Part model, mm, in its own coordinate system. A direction names the side the tool comes from. Round coordinates to 2 decimals unless told otherwise and drop trailing zeros. Order: outer loops, then holes, each group sorted by start corner. A loop starts at its lowest first (then second) coordinate and runs counter-clockwise, first axis right, second up. Notation, with made-up numbers: M 53.5,67 L 93.5,67 A22 ccw 93.5,86 Z; hole C 89.25,-18 d2. An arc over 180 degrees is marked long. Write each question's results on one line, items separated by ' | '. Start each with the question number.
1. Band-saw the part on A-A, the plane y = 0. List the corners of the cut face in (x, z), then the cut area to 3 significant figures.
2. Band-saw the part on D-D, the plane z = 13.5. List the corners of the cut face in (x, y), then the cut area to 3 significant figures.
3. Which spindle directions (+Z, -Z, +X, -X, +Y, -Y) get a long thin tool onto all of the face, cutting with end or side? Do faces 1 (the face through (20.765, 39.923, 49.58)), 2 (the face through (-14.985, -0.66, 29.58)). Say none if no direction does.
4. Two-plate mould, pull along X, no slides. Class faces 3 (the face through (-120, 0, 10)), 4 (the face through (15, -7, 60)), 5 (the face through (120, 0, 10)): +X half, -X half, draft (parallel to the pull), parting line (faces both ways), or undercut.
5. Drop flat-ended pins along their axis: pin 1 Ø12 at (y, z) = (-6.5, 14.5) entering from +X; pin 2 Ø2 at (x, y) = (36, 20) entering from -Z; pin 3 Ø5 at (x, z) = (-15.5, 61) entering from -Y; pin 4 Ø1.5 at (x, z) = (-8.5, 69) entering from +Y. Give the stop position or say it passes through.
6. Band-saw the part on C-C, the plane z = 51.5. List the corners of the cut face in (x, y), then the cut area to 3 significant figures.
7. Probe L1, parallel to Y at x = 0, z = 13; L2, parallel to Y at x = 0, z = 31; L3, parallel to Z at x = -22.5, y = -2. List the from-to ranges inside material, lowest first. Write a range as [from, to].
8. Band-saw the part on B-B, the plane x = -100. List the corners of the cut face in (y, z), then the cut area to 3 significant figures.
Autodesk Fusion 360 part; units mm, degrees
sketch "Sketch1" plane through (0, 0, 0) normal (0, 0, 1) x (1, 0, 0)
  circle A0 centre (0, 0) radius 15
  circle A1 centre (0, 0) radius 35
  circle A2 centre (0, 0) radius 45
  line L0 (-100, -20.9657) -> (-100, -80.0578) construction
  circle A3 centre (-100, 0) radius 12.5
  circle A4 centre (100, 0) radius 12.5
  line L1 (-106, 19.0788) -> (-15, 47.697)
  arc A5 (-106, 19.0788) -> (-106, -19.0788) centre (-100, 0) ccw
  line L2 (-106, -19.0788) -> (-15, -47.697)
  line L3 (106, 19.0788) -> (15, 47.697)
  line L4 (106, -19.0788) -> (15, -47.697)
  arc A6 (-15, -47.697) -> (15, -47.697) centre (0, 0) ccw
  arc A7 (15, 47.697) -> (-15, 47.697) centre (0, 0) ccw
  line L5 (100, -15) -> (100, -80.0578) construction
  line L6 (-100, 50) -> (-100, 80.9539) construction
  arc A8 (100, -20) -> (106, 19.0788) centre (100, 0) ccw
  dimension "d1" = 30
  dimension "d2" = 70
  dimension "d3" = 90
  dimension "d4" = 100
  dimension "d7" = 25
  dimension "d8" = 40
extrude "Extrude1" add sketch "Sketch1" along normal blind 20 contours L1 A5 L2 L3 L4 A6 A7 A8
extrude "Extrude2" add sketch "Sketch1" along normal blind 80 contours A2
extrude "Extrude3" add sketch "Sketch1" along normal blind 60 contours A1
Solution:
1) outline: M -120,0 L -112.5,0 L -112.5,20 L -120,20 Z; M -87.5,0 L -15,0 L -15,60 L -35,60 L -35,80 L -45,80 L -45,20 L -87.5,20 Z; M 15,0 L 87.5,0 L 87.5,20 L 45,20 L 45,80 L 35,80 L 35,60 L 15,60 Z; M 112.5,0 L 120,0 L 120,20 L 112.5,20 Z | area: 6,000 mm^2
2) outline: M -106,-19.08 L -15,-47.7 A50 ccw 15,-47.7 L 106,-19.08 A20 ccw 106,19.08 L 15,47.7 A50 ccw -15,47.7 L -106,19.08 A20 ccw Z; hole C -100,0 d25; hole C 0,0 d30; hole C 100,0 d25 | area: 14,200 mm^2
3) face 1: +Z | face 2: +Z, -Z
4) face 3: -X half | face 4: undercut | face 5: +X half
5) pin 1: x = 119.99 | pin 2: z = 0 | pin 3: y = -43.08 | pin 4: y = 44.33
6) outline: C 0,0 d90; hole C 0,0 d30 | area: 5,650 mm^2
7) L1: [-50, -15], [15, 50] | L2: [-45, -15], [15, 45] | L3: [0, 60]
8) outline: M -20.97,0 L -12.5,0 L -12.5,20 L -20.97,20 Z; M 12.5,0 L 20.97,0 L 20.97,20 L 12.5,20 Z | area: 339 mm^2
